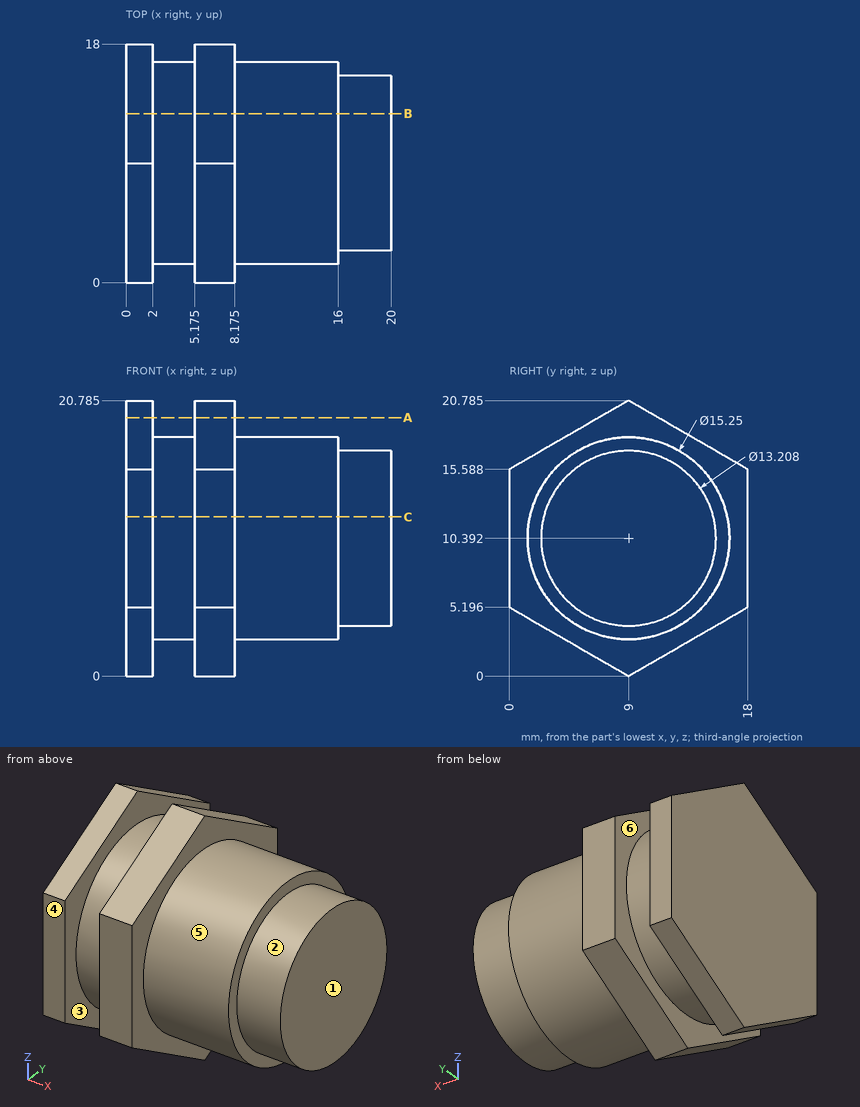
Input: dimensioned drawing with shaded views. Units: mm. Origin: part minimum x, y, z. A direction names the side the tool comes from. Coordinates: 2 decimals unless noted, no trailing zeros. Loops run counter-clockwise (first coordinate to the right, second up) from the corner with the lowest first, then second, coordinate; pieces in that order, holes last.
Q1. Section C-C, the plane z = 12. Return the cut outline in (x, y) (1 decimal), and give its area (3 significant figures).
Results are:
outline: (0, 0) - (2, 0) - (2, 1.5) - (5.2, 1.5) - (5.2, 0) - (8.2, 0) - (8.2, 1.5) - (16, 1.5) - (16, 2.6) - (20, 2.6) - (20, 15.4) - (16, 15.4) - (16, 16.5) - (8.2, 16.5) - (8.2, 18) - (5.2, 18) - (5.2, 16.5) - (2, 16.5) - (2, 18) - (0, 18) - close
area: 305 mm2
Q2. Set-up query: the marked faces 4, 5 and 6. Return all of +Z, -Z, +X, -X, +Y, -Y with unobstructed straight access to the full face (end or side cutting, diameter ignored); none if empty.
Results are:
face 4: +Z, -Z, +X, -X, -Y
face 5: +X
face 6: none
Q3. Contact query for flat-ended pins moving along their axis: pin 1 (1 mm diameter, centred on x = 4, y = 7.5, fed in from -Z); pin 2 (1 mm diameter, centred on x = 17, z = 4, fed in from +Y) (1 decimal); pin 3 (6 mm diameter, centred on x = 2.5, y = 5, fed in from +Z). Output: stop coordinate, or through.
Results are:
pin 1: stops at z = 2.83
pin 2: stops at y = 12
pin 3: stops at z = 20.18
Q4. Section A-A, the plane z = 19.5. Return the cut outline in (x, y) (1 decimal).
Results are:
outline: (0, 6.8) - (2, 6.8) - (2, 11.2) - (0, 11.2) - close; (5.2, 6.8) - (8.2, 6.8) - (8.2, 11.2) - (5.2, 11.2) - close
Q5. Line query: line 1 along X through (y, z) = (14.75, 16) (1 decimal); line 2 along Y through (x, z) = (4.5, 10.25); line 3 along Z through (x, y) = (8.25, 10). Output: solid intervals per line, ascending.
Results are:
line 1: x = 0 to 2, 5.2 to 8.2
line 2: y = 1.38 to 16.62
line 3: z = 2.83 to 17.95
Q6. Section B-B, the plane y = 12.75. Return the cut outline in (x, z) (1 decimal), and give its area (3 significant figures).
Results are:
outline: (0, 2.2) - (2, 2.2) - (2, 3.8) - (5.2, 3.8) - (5.2, 2.2) - (8.2, 2.2) - (8.2, 3.8) - (16, 3.8) - (16, 5) - (20, 5) - (20, 15.8) - (16, 15.8) - (16, 17) - (8.2, 17) - (8.2, 18.6) - (5.2, 18.6) - (5.2, 17) - (2, 17) - (2, 18.6) - (0, 18.6) - close
area: 272 mm2
Q7. Mould query, pull axis X, two halves, no side actions, for the marked faces 1, 2 and 3. Classes: +X half, -X half, draft (parallel to the pull), parting line (faces both ways), or undercut.
Results are:
face 1: +X half
face 2: draft
face 3: undercut
